Can you work these out from the model? Positions are in its coordinate system, mm. A direction names the side the tool comes from. Coordinates: 2 decimals unless noted, no trailing zeros. Write each loop counter-clockwise with the first axis right and the second up, starting at its lowest first coordinate (ties: lowest second). Pieces come first, ordered by that corner, then holes. Notation, with made-up numbers: (84, 42.25) - (89, 42.25) arc R27 cw to (89, 58.25) - close; hole circle Ø9 at (-10, -5.5). An arc over 180 degrees is marked (long way). One line per question, with ' | ' between items. Start each with the question number.
Solid Edge part; units mm, degrees
sketch "Sketch1" plane through (0, 0, 0) normal (0, -1, 0) x (1, 0, 0)
  circle A0 centre (0, 0) radius 19.05
extrude "Hub" add sketch "Sketch1" against normal blind 3.175 and the other way blind 19.05
sketch "Sketch2" plane through (0, -19.05, 0) normal (0, -1, 0) x (1, 0, 0)
  line L0 (-10.1719, 16.107) -> (96.9811, 83.776)
  arc A0 (109.6445, 66.3463) -> (96.9811, 83.776) centre (102.7452, 74.6487) ccw
  line L1 (12.1754, -14.6514) -> (109.6445, 66.3463)
  arc A1 (-10.1719, 16.107) -> (12.1754, -14.6514) centre (0, 0) ccw
  circle A2 centre (102.7452, 74.6487) radius 4.445
extrude "Crank_Arm" add sketch "Sketch2" along normal blind 6.35
fillet "Round_8" radius 3.175 4 edges at (43.4046, -25.4, 49.9415) (-15.4118, -25.4, -11.1973) (111.4785, -25.4, 80.9939) (111.4785, -19.05, 80.9939)
sketch "Sketch3" plane through (33.1969, -25.4, 47.2451) normal (0, -1, 0) x (0.8455, 0, 0.534)
  circle A0 centre (-53.2952, -22.2206) radius 10.16
extrude "ExtrudedCutout_1" cut sketch "Sketch3" against normal blind 12.7
sketch "Sketch4" plane through (0, -12.7, 0) normal (0, -1, 0) x (0, 0, 1)
  line L0 (-4.445, -4.445) -> (4.445, -4.445)
  line L1 (4.445, -4.445) -> (4.445, 4.445)
  line L2 (4.445, 4.445) -> (-4.445, 4.445)
  line L3 (-4.445, 4.445) -> (-4.445, -4.445)
extrude "Cutout1" cut sketch "Sketch4" against normal through all
properties part number "8-12" material "Aluminum, 7075-T6"
(1) Which directions (+Z, -Z, +X, -X, +Y, -Y) give clear straight access to the entire face, cutting with the end or side of a thin tool? Please do faces 1 (the face through (43.14, -20, 48.7)), 2 (the face through (-4.445, -5, 0)), 3 (the face through (-15.12, -9.7, -11.59)), 4 (the face through (5, 3.175, 0)), 5 (the face through (3.44, -19.14, -9.56)).
(2) I'm going to push flat-ended pins straight in: pin 1 (1.5 mm diameter, centred on y = -10.5, z = -7, fed in from -X); pin 2 (6 mm diameter, centred on x = 2, z = 3.5, fed in from -Y); pin 3 (4.5 mm diameter, centred on x = 1, y = -2, fed in from +Z); pin 4 (4 mm diameter, centred on y = -17, z = 48, fed in from -X). Where does each tip first touch, or does it pass through?
(3) If we section it at B-B on y = -15.5: List the corners of the cut face in (x, z) for me, plus the area to 3 significant figures.
(4) If I drill on probe 1 along Y at (x, z) = (19, 11.5); probe 2 along Z at (x, y) = (-0.5, -19.75); probe 3 along X at (y, z) = (-16, 5), over which ranges is the centre line in solid material (lowest first)?
(5) If we section it at A-A on y = -9.25: List the corners of the cut face in (x, z) for me (3 decimals), plus the area to 3 significant figures.
(6) If we mould it in two halves opening along X, with no side actions, what happens to faces 6 (the face through (106.85, -22.18, 76.35)), 7 (the face through (59.65, -24.45, 25.98)), 8 (the face through (52, -19.05, 38))? For each: +X half, -X half, draft (parallel to the pull), parting line (faces both ways), or undercut.
Values:
1) face 1: +Z, -X, +Y | face 2: +Y, -Y | face 3: +Y | face 4: +Z, -Z, +X, -X, +Y | face 5: -Y
2) pin 1: x = -18 | pin 2: y = -12.7 | pin 3: z = 19.05 | pin 4: through
3) outline: circle Ø38.1 at (0, 0); hole circle Ø20.32 at (0, 0) | area: 816 mm2
4) probe 1: -25.4 to -19.05 | probe 2: -19.04 to -10.15, 10.15 to 20.81 | probe 3: -18.38 to -8.84, 8.85 to 18.38
5) outline: circle Ø38.1 at (0, 0); hole (-4.445, -4.445) - (4.445, -4.445) - (4.445, 4.445) - (-4.445, 4.445) - close | area: 1,060 mm2
6) face 6: undercut | face 7: +X half | face 8: draft
